Could you check a few things on this drawing? It's one solid part, dimensions in mm from its lowest x, y, z. A direction names the side the tool comes from. Give positions to 0.01 mm unless a question says otherwise; leave off trailing zeros. Loops run counter-clockwise (first coordinate to the right, second up) from the corner with the lowest first, then second, coordinate; pieces in that order, holes last. Notation, with made-up numbers: (25, 38.25) - (36, 38.25) arc R22 ccw to (36, 52.25) - close; hole circle Ø1 at (76.25, -38.75). An arc over 180 degrees is marked (long way). One line per item, written item: value. Start each with the question number.
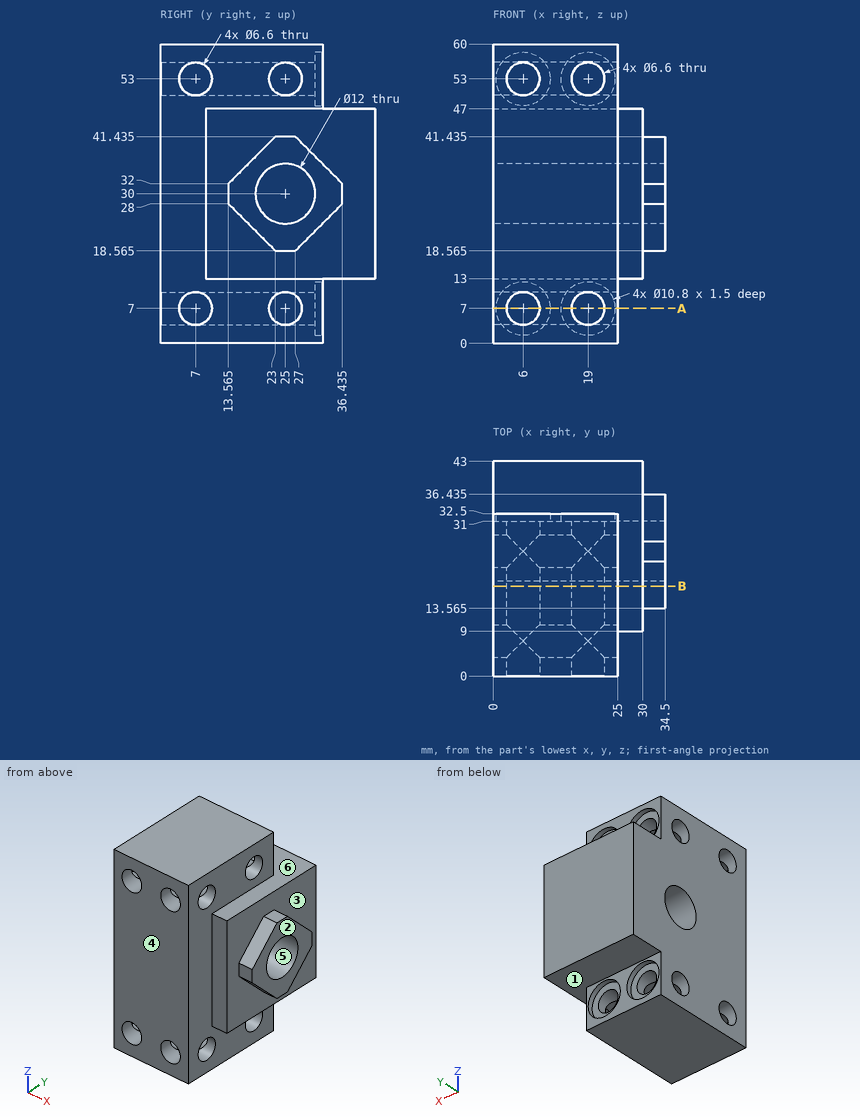
(1) If we section it at B-B on y = 18: List the corners of the cut face in (x, z) for me (3 decimals), plus the area to 3 significant figures.
(2) Please list where these lines run through material, in increasing order: probe 1 along X at (y, z) = (32, 7); probe 2 along Z at (x, y) = (6, 2.25); probe 3 along X at (y, z) = (3.5, 53). Write a range as from..to.
(3) If we mould it in two halves opening along Y, with no side actions, what happens to the marked faces 4, 5 and 6? For each: pulls with the +Y half, pulls with the -Y half, needs draft (parallel to the pull), parting line crosses it, or undercut.
(4) Will these pins go through, and if not, where does the flat tip stop? pin 1 (6 mm diameter, centred on x = 19, z = 7, fed in from -Y); pin 2 (5.5 mm diameter, centred on x = 20.5, z = 7.5, fed in from +Y); pin 3 (3 mm diameter, centred on x = 32.5, y = 25, fed in from +Z) (3 decimals); pin 4 (4 mm diameter, centred on x = 30.5, y = 15, fed in from -Z).
(5) For the marked faces 1, 2 and 3, which set-ups out of +Z, -Z, +X, -X, +Y, -Y let a thin tool reach every point of the face, with its end or its side?
(6) If we section it at A-A on z = 7: Give the number of separate pieces and of enclosed holes in the cut face, plus the area to 3 significant figures.
Found:
1. outline: (0, 0) - (25, 0) - (25, 13) - (30, 13) - (30, 23.565) - (34.5, 23.565) - (34.5, 36.435) - (30, 36.435) - (30, 47) - (25, 47) - (25, 60) - (0, 60) - close; hole circle Ø6.6 at (6, 7); hole circle Ø6.6 at (6, 53); hole circle Ø6.6 at (19, 7); hole circle Ø6.6 at (19, 53)
1. area: 1,590 mm^2
2. probe 1: 0..0.6, 11.4..13.6, 24.4..25
2. probe 2: 0..3.7, 10.3..49.7, 56.3..60
2. probe 3: 0..2.7, 9.3..15.7, 22.3..25
3. face 4: pulls with the -Y half
3. face 5: undercut
3. face 6: needs draft
4. pin 1: through
4. pin 2: y = 31
4. pin 3: z = 41.435
4. pin 4: z = 13
5. face 1: -Z, +X, +Y
5. face 2: +Z, -Z, +X, +Y, -Y
5. face 3: +X
6. separate pieces: 9
6. enclosed holes: 0
6. area: 215 mm^2
